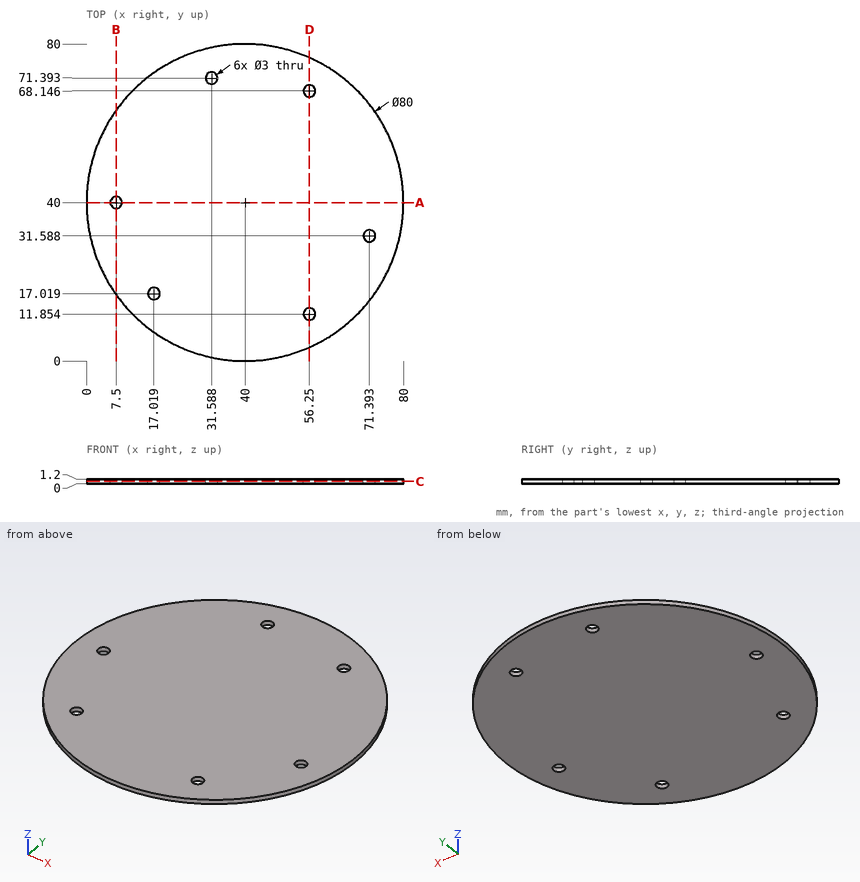
Source: three-view drawing plus pictorial views. Frame: mm from the lowest corner of the part. Coordinates: 2 decimals unless noted, no trailing zeros. Loops run counter-clockwise (first coordinate to the right, second up) from the corner with the lowest first, then second, coordinate; pieces in that order, holes last. Notation, with made-up numbers: (7.25, 40) - (23.25, 40) arc R14 cw to (23.25, 52) - close; hole circle Ø7 at (-21.75, 29.25). An arc over 180 degrees is marked (long way). One line per item, written item: value. Start each with the question number.
1. Contact query for flat-ended pins moving along their axis: P1, Ø3.5, axis at x = 56.25, y = 68.15, coming from the -Z side; P2, Ø2.5, axis at x = 31.59, y = 71.39, coming from the +Z side. Output: stop coordinate, or through.
2. Section A-A (y = 40). Return the cut outline in (x, z).
3. Ray query, L1, parallel to X at y = 68.5, z = 0.15 (1 decimal); L2, parallel to X at y = 17.5, z = 0.5; L3, parallel to Y at x = 17, z = 1 (1 decimal). Return the intervals inside material, ascending.
4. Section C-C (z = 0.6). Return the cut outline in (x, y), and give its area (3 significant figures).
5. Section D-D (x = 56.25). Return the cut outline in (y, z).
6. Section B-B (x = 7.5). Return the cut outline in (y, z).
Verdict:
1. P1: stops at z = 0
1. P2: passes through
2. outline: (0, 0) - (6, 0) - (6, 1.2) - (0, 1.2) - close; (9, 0) - (80, 0) - (80, 1.2) - (9, 1.2) - close
3. L1: x = 11.9 to 54.8, 57.7 to 68.1
3. L2: x = 6.93 to 15.6, 18.44 to 73.07
3. L3: y = 7.3 to 15.5, 18.5 to 72.7
4. outline: circle Ø80 at (40, 40); hole circle Ø3 at (7.5, 40); hole circle Ø3 at (17.02, 17.02); hole circle Ø3 at (31.59, 71.39); hole circle Ø3 at (56.25, 11.85); hole circle Ø3 at (56.25, 68.15); hole circle Ø3 at (71.39, 31.59)
4. area: 4,980 mm2
5. outline: (3.45, 0) - (10.35, 0) - (10.35, 1.2) - (3.45, 1.2) - close; (13.35, 0) - (66.65, 0) - (66.65, 1.2) - (13.35, 1.2) - close; (69.65, 0) - (76.55, 0) - (76.55, 1.2) - (69.65, 1.2) - close
6. outline: (16.68, 0) - (38.5, 0) - (38.5, 1.2) - (16.68, 1.2) - close; (41.5, 0) - (63.32, 0) - (63.32, 1.2) - (41.5, 1.2) - close
